Study the drawing (mm; zero at the part's minimum x, y, z) and answer. A direction names the side the tool comes from. Give positions to 0.01 mm unless a question says otherwise; leave off trailing zeros. Loops run counter-clockwise (first coordinate to the right, second up) from the corner with the lowest first, then second, coordinate; pieces in that order, holes last. Notation, with made-up numbers: (28.5, 86.25) - (71.5, 86.25) arc R21 ccw to (71.5, 99.25) - close; hole circle Ø10 at (61.25, 15.5). An arc over 180 degrees is marked (long way). Write item = value, one per line. Start each with the question number.
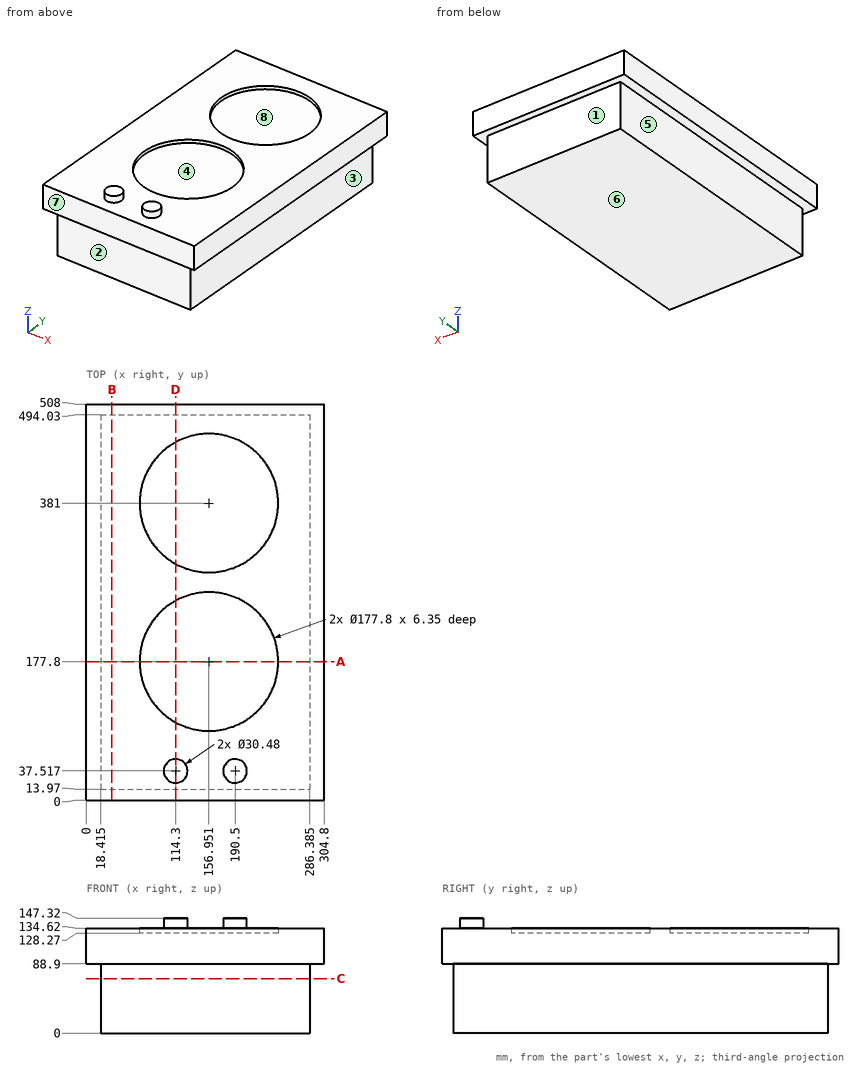
1. Given P1, Ø10, axis at y = 323.5, z = 67, coming from the -X side (3 decimals); P2, Ø8, axis at x = 127.5, y = 299, coming from the +Z side; P3, Ø8, axis at y = 374, z = 59, coming from the +X side (3 decimals), each flat-ended and moving along its own axis, determine where each tip first touches the part or whether it passes through.
2. A cutting plane is placed at B-B on x = 32.5. Give the vertices of the cut face in (y, z), and give its area (3 significant figures).
3. A cutting plane is placed at D-D on x = 114.3. Give the vertices of the cut face in (y, z).
4. A cutting plane is placed at C-C on z = 70. Give the vertices of the cut face in (x, y) (1 decimal), and give its area (3 significant figures).
5. A tool of negligible diameter and unlimited length cuts with its end or side. For the marked faces 1, 2, 3, 4 and 5, from which of +Z, -Z, +X, -X, +Y, -Y can it reach the whole face along a straight path? Write none if from no direction.
6. A cutting plane is placed at A-A on y = 177.8. Give the vertices of the cut face in (x, z) (1 decimal).
7. For a pull along Y with two mould halves and no side action, classify the marked faces 6, 7 and 8 as released by +Y, released by -Y, zero draft, split by the parting line, or undercut.
8. Consider line 1 along X through (y, z) = (177, 133) (1 decimal); line 2 along X through (y, z) = (186.5, 63) (1 decimal); line 3 along Y through (x, z) = (232.5, 79). Determine where each line is inside the solid, lowest interval first. Write a range as [from, to].
Reply:
q1.P1 = 18.415
q1.P2 = 134.62
q1.P3 = 286.385
q2.outline = (0, 88.9) - (13.97, 88.9) - (13.97, 0) - (494.03, 0) - (494.03, 88.9) - (508, 88.9) - (508, 134.62) - (0, 134.62) - close
q2.area = 65,900 mm^2
q3.outline = (0, 88.9) - (13.97, 88.9) - (13.97, 0) - (494.03, 0) - (494.03, 88.9) - (508, 88.9) - (508, 134.62) - (459, 134.62) - (459, 128.27) - (303, 128.27) - (303, 134.62) - (255.8, 134.62) - (255.8, 128.27) - (99.8, 128.27) - (99.8, 134.62) - (52.76, 134.62) - (52.76, 147.32) - (22.28, 147.32) - (22.28, 134.62) - (0, 134.62) - close
q4.outline = (18.4, 14) - (286.4, 14) - (286.4, 494) - (18.4, 494) - close
q4.area = 129,000 mm^2
q5.face_1 = -Z, +X, -X, +Y
q5.face_2 = -Z, +X, -X, -Y
q5.face_3 = -Z, +X, +Y, -Y
q5.face_4 = +Z
q5.face_5 = -Z, -X, +Y, -Y
q6.outline = (0, 88.9) - (18.4, 88.9) - (18.4, 0) - (286.4, 0) - (286.4, 88.9) - (304.8, 88.9) - (304.8, 134.6) - (245.9, 134.6) - (245.9, 128.3) - (68.1, 128.3) - (68.1, 134.6) - (0, 134.6) - close
q7.face_6 = zero draft
q7.face_7 = released by -Y
q7.face_8 = undercut
q8.line_1 = [0, 68.1], [245.8, 304.8]
q8.line_2 = [18.4, 286.4]
q8.line_3 = [13.97, 494.03]
